Check sheet for the modelled part. Datum: model origin and axes. Units: mm. A direction names the side the tool comes from. Round coordinates to 2 decimals unless told otherwise and drop trailing zeros. Write each loop counter-clockwise with the first axis right and the second up, starting at its lowest first coordinate (ties: lowest second). Pieces come first, ordered by that corner, then holes. Notation, with made-up numbers: (-20, 5) -> (39, 5) arc R14 ccw to (39, 32) -> close; hole circle Ø2 at (-38, 80). An arc over 180 degrees is marked (long way). Write item = value, one per line.
from build123d import *

# Parameters (mm, degrees)
BOX007_W               = 3
BOX007_H               = 6
BOX007_DEPTH           = 5
BOX008_W               = 3
BOX008_H               = 10
BOX008_DEPTH           = 10
BOX008_PLACEMENT_ANGLE = 45
BOX009_W               = 3
BOX009_H               = 10
BOX009_DEPTH           = 10
BOX009_PLACEMENT_ANGLE = 45
BOX006_W               = 3
BOX006_H               = 6
BOX006_DEPTH           = 5
BOX005_W               = 12
BOX005_H               = 0.5
BOX005_DEPTH           = 6.8
BOX004_W               = 22
BOX004_H               = 29
BOX004_DEPTH           = 0.6
BOX001_W               = 10
BOX001_H               = 15
BOX001_DEPTH           = 6
BOX002_W               = 10
BOX002_H               = 10
BOX002_DEPTH           = 6
BOX003_W               = 13
BOX003_H               = 4
BOX003_DEPTH           = 6
BOX_W                  = 21
BOX_H                  = 1.8
BOX_DEPTH              = 6.8
ARRAY_X_COUNT          = 2
ARRAY_X_PITCH          = 34
SKETCH001_R            = 0.6
EXTRUDE_DEPTH          = 6.8


with BuildPart() as wire02:
    # Box007 → Box007 (new body)
    with BuildSketch(Plane(origin=(14, 8, 3), x_dir=(1, 0, 0), z_dir=(0, 0, 1))):
        with Locations((1.5, 3)):
            Rectangle(BOX007_W, BOX007_H)
    extrude(amount=BOX007_DEPTH)


with BuildPart() as wire11:
    # Box008 → Box008 (new body)
    with BuildSketch(Plane.XY):
        with Locations((1.5, 5)):
            Rectangle(BOX008_W, BOX008_H)
    extrude(amount=BOX008_DEPTH)


with BuildPart() as wire11_1:
    # Box008 placement: moved
    add(wire11.part.moved(Location((-14, 14, 3))).rotate(Axis((-14, 14, 3), (0, 0, 1)), BOX008_PLACEMENT_ANGLE))


with BuildPart() as wire12:
    # Box009 → Box009 (new body)
    with BuildSketch(Plane.XY):
        with Locations((1.5, 5)):
            Rectangle(BOX009_W, BOX009_H)
    extrude(amount=BOX009_DEPTH)


with BuildPart() as wire12_1:
    # Box009 placement: moved
    add(wire12.part.moved(Location((12, 16, 3))).rotate(Axis((12, 16, 3), (0, 0, -1)), BOX009_PLACEMENT_ANGLE))


with BuildPart() as wires:
    # Box006 → Box006 (new body)
    with BuildSketch(Plane(origin=(-17, 8, 3), x_dir=(1, 0, 0), z_dir=(0, 0, 1))):
        with Locations((1.5, 3)):
            Rectangle(BOX006_W, BOX006_H)
    extrude(amount=BOX006_DEPTH)

    # Fusion004: union wire02, wire11, wire12
    add(wire02.part)
    add(wire11_1.part)
    add(wire12_1.part)


with BuildPart() as box005:
    # Box005 → Box005 (new body)
    with BuildSketch(Plane(origin=(11, -35, 0), x_dir=(1, 0, 0), z_dir=(0, 0, 1))):
        with Locations((6, 0.25)):
            Rectangle(BOX005_W, BOX005_H)
    extrude(amount=BOX005_DEPTH)


with BuildPart() as box004:
    # Box004 → Box004 (new body)
    with BuildSketch(Plane(origin=(-11, -31, 0), x_dir=(1, 0, 0), z_dir=(0, 0, 1))):
        with Locations((11, 14.5)):
            Rectangle(BOX004_W, BOX004_H)
    extrude(amount=BOX004_DEPTH)


with BuildPart() as obj1:
    # Box001 → Box001 (new body)
    with BuildSketch(Plane(origin=(-5, 0, 2.2), x_dir=(1, 0, 0), z_dir=(0, 0, 1))):
        with Locations((5, 7.5)):
            Rectangle(BOX001_W, BOX001_H)
    extrude(amount=BOX001_DEPTH)


with BuildPart() as pin:
    # Box002 → Box002 (new body)
    with BuildSketch(Plane(origin=(-5, -2, 1.4), x_dir=(1, 0, 0), z_dir=(0, 0, 1))):
        with Locations((5, 5)):
            Rectangle(BOX002_W, BOX002_H)
    extrude(amount=BOX002_DEPTH)


with BuildPart() as solder:
    # Box003 → Box003 (new body)
    with BuildSketch(Plane(origin=(-6.5, 0, 2), x_dir=(1, 0, 0), z_dir=(0, 0, 1))):
        with Locations((6.5, 2)):
            Rectangle(BOX003_W, BOX003_H)
    extrude(amount=BOX003_DEPTH)


with BuildPart() as array:
    # Box → Box (new body)
    with BuildSketch(Plane(origin=(-10.5, 0, 0), x_dir=(1, 0, 0), z_dir=(0, 0, 1))):
        with Locations((10.5, 0.9)):
            Rectangle(BOX_W, BOX_H)
    extrude(amount=BOX_DEPTH)

    # Fusion: union obj1, pin, solder
    add(obj1.part)
    add(pin.part)
    add(solder.part)


with BuildPart() as array_1:
    # Fusion placement: moved
    add(array.part.moved(Location((-17, -33.5, 0))))

    # Array X: Array ×2


with BuildPart() as array_2:
    add(array_1.part)
    with Locations(*[(i * ARRAY_X_PITCH, 0, 0) for i in range(1, ARRAY_X_COUNT)]):
        add(array_1.part)


with BuildPart() as cut001:
    # Sketch001 → Extrude (new body)
    with BuildSketch(Plane.XY):
        with BuildLine():
            ThreePointArc((32, 0), (0, 32), (-32, 0))
            Line((-32, 0), (-32, -30.035479))
            ThreePointArc((-32, -30.035479), (-30.545926, -33.545926), (-27.035479, -35))
            Line((-27.035479, -35), (27.049982, -35))
            ThreePointArc((27.049982, -35), (30.550173, -33.550173), (32, -30.049982))
            Line((32, -30.049982), (32, 0))
        make_face()
        with Locations((-27, -25)):
            Circle(SKETCH001_R, mode=Mode.SUBTRACT)
        with Locations((27, -25)):
            Circle(SKETCH001_R, mode=Mode.SUBTRACT)
        with Locations((-24, 14)):
            Circle(SKETCH001_R, mode=Mode.SUBTRACT)
        with Locations((24, 14)):
            Circle(SKETCH001_R, mode=Mode.SUBTRACT)
        with BuildLine():
            Line((-28.283536, 10.002079), (-11.283536, 10.002079))
            Line((-9.821695, 10.002079), (-11.283536, 10.002079))
            ThreePointArc((-9.821695, 10.002079), (-9.651432, 10.072604), (-9.580907, 10.242867))
            Line((-9.580907, 20.003923), (-9.580907, 10.242867))
            Line((-9.580907, 20.003923), (9.580907, 20.003923))
            Line((9.580907, 20.003923), (9.580907, 10.20069))
            ThreePointArc((9.580907, 10.20069), (9.639688, 10.058781), (9.781597, 10))
            Line((9.781597, 10), (10.999997, 10))
            Line((10.999997, 10), (27.999997, 10))
            ThreePointArc((29.732135, 0), (29.2959, 5.074453), (27.999997, 10))
            Line((29.732135, -5), (29.732135, 0))
            Line((29.732135, -5), (11.449554, -5))
            ThreePointArc((10.998979, -4.549425), (11.130949, -4.86803), (11.449554, -5))
            Line((10.998979, -2.047611), (10.998979, -4.549425))
            ThreePointArc((10.998979, -2.047611), (10.951968, -1.934117), (10.838474, -1.887106))
            Line((9.826898, -1.887106), (10.838474, -1.887106))
            ThreePointArc((9.826898, -1.887106), (9.69096, -1.943413), (9.634653, -2.079351))
            Line((9.634653, -4.996077), (9.634653, -2.079351))
            Line((9.634653, -4.996077), (6.387418, -4.996077))
            ThreePointArc((6.387418, -4.996077), (6.154439, -5.09258), (6.057936, -5.325559))
            Line((6.057936, -5.325559), (6.057936, -6.717126))
            ThreePointArc((6.057936, -6.717126), (6.15523, -6.952016), (6.390121, -7.049311))
            Line((6.390121, -7.049311), (29.401567, -7.049311))
            ThreePointArc((30.016101, -7.663845), (29.836108, -7.229304), (29.401567, -7.049311))
            Line((30.016101, -7.663845), (30.016101, -11.257143))
            Line((30.016101, -17.879205), (30.016101, -11.257143))
            ThreePointArc((24.990135, -22.90517), (28.544029, -21.433099), (30.016101, -17.879205))
            Line((24.990135, -22.90517), (9.5, -22.90517))
            Line((9.5, -30), (9.5, -22.90517))
            Line((9.5, -30), (-9.5, -30))
            Line((-9.5, -30), (-9.5, -22.889064))
            Line((-24.982737, -22.889064), (-9.5, -22.889064))
            ThreePointArc((-30, -17.879205), (-28.530028, -21.424329), (-24.982737, -22.889064))
            Line((-30, -11.257325), (-30, -17.879205))
            Line((-30, -11.257325), (-30, -7.602077))
            ThreePointArc((-29.400597, -7.002674), (-29.824439, -7.178235), (-30, -7.602077))
            Line((-29.400597, -7.002674), (-6.477289, -7.002674))
            ThreePointArc((-6.477289, -7.002674), (-6.211158, -6.892439), (-6.100923, -6.626308))
            Line((-6.100923, -5.308623), (-6.100923, -6.626308))
            ThreePointArc((-6.100923, -5.308623), (-6.191681, -5.089514), (-6.41079, -4.998756))
            Line((-9.365347, -4.998756), (-6.41079, -4.998756))
            Line((-9.365347, -2.082029), (-9.365347, -4.998756))
            ThreePointArc((-9.365347, -2.082029), (-9.461983, -1.848728), (-9.695285, -1.752091))
            Line((-10.706861, -1.752091), (-9.695285, -1.752091))
            ThreePointArc((-10.706861, -1.752091), (-10.915611, -1.838558), (-11.002079, -2.047309))
            Line((-11.002079, -4.549979), (-11.002079, -2.047309))
            ThreePointArc((-11.450021, -4.997921), (-11.133278, -4.866722), (-11.002079, -4.549979))
            Line((-11.450021, -4.997921), (-30, -4.997921))
            Line((-30, -4.997921), (-30, 0))
            ThreePointArc((-28.283536, 10.002079), (-29.56777, 5.074146), (-30, 0))
        make_face(mode=Mode.SUBTRACT)
        with BuildLine():
            ThreePointArc((11.150322, 26.770699), (-0.151775, 28.999603), (-11.429923, 26.652521))
            Line((-9.58106, 23.01514), (-11.429923, 26.652521))
            ThreePointArc((-9.58106, 23.01514), (-8.322568, 21.651708), (-6.53689, 21.147623))
            Line((-6.53689, 21.147623), (6.776723, 21.147623))
            ThreePointArc((6.776723, 21.147623), (8.461354, 21.657225), (9.58106, 23.01514))
            Line((11.150322, 26.770699), (9.58106, 23.01514))
        make_face(mode=Mode.SUBTRACT)
        with BuildLine():
            ThreePointArc((-16.458256, 25.678314), (-21.184389, 21.942462), (-25.084031, 17.350544))
            Line((-24.167702, 16.028793), (-25.084031, 17.350544))
            ThreePointArc((-15.677322, 24.397163), (-20.357158, 20.653961), (-24.167702, 16.028793))
            Line((-15.677322, 24.397163), (-16.458256, 25.678314))
        make_face(mode=Mode.SUBTRACT)
        with BuildLine():
            ThreePointArc((25.084031, 17.350544), (21.184389, 21.942462), (16.458256, 25.678314))
            Line((16.458256, 25.678314), (15.677322, 24.397163))
            ThreePointArc((24.167702, 16.028793), (20.357158, 20.653961), (15.677322, 24.397163))
            Line((25.084031, 17.350544), (24.167702, 16.028793))
        make_face(mode=Mode.SUBTRACT)
        with BuildLine():
            Line((-11.580907, 19.737881), (-11.580907, 12))
            Line((-19.119635, 12), (-11.580907, 12))
            ThreePointArc((-19.940526, 13.375741), (-19.920653, 12.454819), (-19.119635, 12))
            Line((-19.940526, 13.375741), (-13.824918, 24.709109))
            ThreePointArc((-12.975828, 24.620182), (-13.370592, 24.948999), (-13.824918, 24.709109))
            Line((-12.975828, 24.620182), (-11.620684, 20.014015))
            ThreePointArc((-11.580907, 19.737881), (-11.590902, 19.877373), (-11.620684, 20.014015))
        make_face(mode=Mode.SUBTRACT)
        with BuildLine():
            Line((12.975828, 24.620182), (11.620684, 20.014015))
            ThreePointArc((11.620684, 20.014015), (11.590902, 19.877373), (11.580907, 19.737881))
            Line((11.580907, 19.737881), (11.580907, 12))
            Line((19.119635, 12), (11.580907, 12))
            ThreePointArc((19.119635, 12), (19.920653, 12.454819), (19.940526, 13.375741))
            Line((13.824918, 24.709109), (19.940526, 13.375741))
            ThreePointArc((13.824918, 24.709109), (13.370592, 24.948999), (12.975828, 24.620182))
        make_face(mode=Mode.SUBTRACT)
    extrude(amount=EXTRUDE_DEPTH)

    # Cut: cut Array
    add(array_2.part, mode=Mode.SUBTRACT)

    # Fusion001: union Box004
    add(box004.part)

    # Fusion003: union Box005
    add(box005.part)

    # Cut001: cut wires
    add(wires.part, mode=Mode.SUBTRACT)


solid = cut001.part
(1) Sectioned sample at A-A on x = 0. Enter the section's corners in (y, z).
Worked answers:
outline = (-35, 0) -> (-2, 0) -> (-2, 0.6) -> (-30, 0.6) -> (-30, 6.8) -> (-35, 6.8) -> close; (20, 0) -> (21.15, 0) -> (21.15, 6.8) -> (20, 6.8) -> close; (29, 0) -> (32, 0) -> (32, 6.8) -> (29, 6.8) -> close
(2) Release check for a two-part mould opening along X. For faces 1 (the flat face through (-10, -4, 6.8)), 2 (the cylindrical face through (28.505, -21.472, 3.352)) record: pulls with the +X half, pulls with the -X half, needs draft (parallel to the pull), parting line crosses it, or undercut.
Worked answers:
face_1 = needs draft
face_2 = undercut
(3) Sectioned sample at C-C on z = 5.5. Count the separate pieces of the cut face and the enclosed holes in it, then the cut area to 3 significant figures.
Worked answers:
separate_pieces = 1
enclosed_holes = 5
area = 1,020 mm²
(4) Material ranges on L1, parallel to X at y = -10.5, z = 5.25; L2, parallel to Y at x = -27, z = 5; L3, parallel to Y at x = 8.5, z = 1.5, recorded low to high. Write a range as [from, to].
Worked answers:
L1 = [-32, -30], [30.02, 32]
L2 = [-35, -33.5], [-31.7, -25.6], [-24.4, -22.47], [-7, -5], [10, 17.18]
L3 = [-35, -33.5], [-31.7, -30], [-7.05, -5], [20, 21.68], [27.73, 30.85]
(5) Go/stop test with flat-tipped pins: P1, Ø1.2, axis at x = -11.5, y = -30, coming from the +Z side; P2, Ø4, axis at x = 13, z = 2, coming from the +Y side; P3, Ø1.6, axis at x = -19.5, y = -34.5, coming from the +Z side; P4, Ø1, axis at x = 4, y = 18, coming from the +Z side. Record where each tip stops, or that it passes through.
Worked answers:
P1 = 6.8
P2 = 30.05
P3 = 1.4
P4 = through
(6) Access from +Z, -Z, +X, -X, +Y, -Y to the whole of each face (thin tool, end or side, straight path). Record for faces 3 (the flat face through (11.581, 16, 3)), 4 (the flat face through (-17.2, 21.44, 4.87)), 5 (the flat face through (-12, -26, 4)).
Worked answers:
face_3 = +Z, -Z
face_4 = +Z
face_5 = +Z, -Y
(7) Sectioned sample at B-B on y = -17. Enter the section's corners in (x, z), then the cut area to 3 significant figures.
Worked answers:
outline = (-32, 0) -> (-30, 0) -> (-30, 6.8) -> (-32, 6.8) -> close; (-11, 0) -> (11, 0) -> (11, 0.6) -> (-11, 0.6) -> close; (30.02, 0) -> (32, 0) -> (32, 6.8) -> (30.02, 6.8) -> close
area = 40.3 mm²
